Geometry check sheet. Reference: the model listing, model coordinates, mm. Give positions to 0.01 mm unless a question says otherwise; leave off trailing zeros.
1. Go/stop test with flat-tipped pins: pin 1 Ø7 at (x, y) = (47.4, 254.8) entering from +Z; pin 2 Ø5 at (x, y) = (127.4, 254.8) entering from +Z. Record where each tip stops, or that it passes through.
2. Release check for a two-part mould opening along Y. For faces 1 (the conical face through (47.7, 257.09, -2.17)), 2 (the flat face through (75, 304.8, -3)), 3 (the flat face through (152.4, 150, -3)) record: +Y half, -Y half, draft (parallel to the pull), parting line (faces both ways), or undercut.
3. Material ranges on L1, parallel to X at y = 254.8, z = -5.4; L2, parallel to Y at x = 47.4, z = -4.75; L3, parallel to Y at x = 147.4, z = -1.25, recorded low to high.
from build123d import *

# Parameters (mm, degrees)
F0_W           = 152.4
F0_H           = 304.8
F1_DEPTH       = 6.35
F3_D           = 4.4
F3_CSINK_D     = 8.96
F3_CSINK_ANGLE = 90
F5_D           = 3.3


with BuildPart() as f1:
    # F0 (on Top) → F1 (new body)
    with BuildSketch(Plane.XY):
        with Locations((76.2, 152.4)):
            Rectangle(F0_W, F0_H)
    extrude(amount=-F1_DEPTH)

    # F3 (through all)
    with Locations(Plane.XY):
        with Locations((127.4, 254.8), (47.4, 254.8)):
            CounterSinkHole(F3_D / 2, F3_CSINK_D / 2, counter_sink_angle=F3_CSINK_ANGLE)

    # F5 (through all)
    with Locations(Plane.XY):
        with Locations((147.4, 246.8), (147.4, 188.8)):
            Hole(F5_D / 2)


solid = f1.part
Result:
1. pin 1: stops at z = -0.98
1. pin 2: stops at z = -1.98
2. face 1: undercut
2. face 2: +Y half
2. face 3: draft
3. L1: x = 0 to 45.2, 49.6 to 125.2, 129.6 to 152.4
3. L2: y = 0 to 252.6, 257 to 304.8
3. L3: y = 0 to 187.15, 190.45 to 245.15, 248.45 to 304.8
